CAD build for the part. Positions are in the model's coordinates, mm. A direction names the side the tool comes from. Give positions to 0.01 mm unless a question says otherwise; leave off trailing zeros. Order: outer loops, then holes, each group sorted by start corner. A loop starts at its lowest first (then second) coordinate and runs counter-clockwise, first axis right, second up.
Item 1: Band-saw the part on A-A on y = 4. Give the cut face in (x, z).
Item 2: Which spindle directions (+Z, -Z, +X, -X, +Y, -Y) get a long thin tool onto all of the face, cutting with end or side? Do faces 1 (the flat face through (-1, -5, 27.006)), 2 (the flat face through (-1, -6, 5)), 3 (the flat face through (-1, 18, 18)). Say none if no direction does.
Item 3: Flat gauge pins, fed straight in: P1, Ø8.5, axis at x = 1.5, z = 19, coming from the -Y side; P2, Ø11, axis at x = 20, z = 3.5, coming from the -Y side. Where does each tip first touch, or does it go through?
Item 4: Band-saw the part on C-C on y = -9. Give the cut face in (x, z).
Item 5: Band-saw the part on B-B on x = -20. Give the cut face in (y, z).
Item 6: Two-plate mould, pull along Z, no slides. Class faces 4 (the flat face through (-1, 0, 37)), 5 (the flat face through (65, 12, 22)), 6 (the flat face through (-1, 1, 10.006)): released by +Z, released by -Z, zero draft, split by the parting line, or undercut.
Item 7: Wall check: L1, parallel to Z at x = 2, y = 3.5; L2, parallel to Y at x = -53.5, z = 2; L3, parallel to Z at x = -49.5, y = -10.5. Give the ranges that are in metal, low to high.
Item 8: Band-saw the part on D-D on z = 22. Give the cut face in (x, y), plus the area to 3 significant figures.
```python
from build123d import *

# Parameters (mm, degrees)
SKETCH_2_W          = 130
SKETCH_2_H          = 36
EXTRUDE_1_DEPTH     = 37
CUT_EXTRUDE_START   = -18
SKETCH_4_W          = 130
SKETCH_4_H          = 17
CUT_EXTRUDE_1_DEPTH = 26
SKETCH_5_W          = 130
SKETCH_5_H          = 12
CUT_EXTRUDE_2_DEPTH = 12


with BuildPart() as part:
    # 스케치2 → 보스-돌출1 (new body)
    with BuildSketch(Plane.XY):
        Rectangle(SKETCH_2_W, SKETCH_2_H)
    extrude(amount=EXTRUDE_1_DEPTH)

    # 스케치4 → 컷-돌출1 (cut)
    with BuildSketch(Plane(origin=(0, 0, 0), x_dir=(1, 0, 0), z_dir=(0, 1, 0)).offset(CUT_EXTRUDE_START)):
        with Locations((0, -18.50644362)):
            Rectangle(SKETCH_4_W, SKETCH_4_H)
    extrude(amount=CUT_EXTRUDE_1_DEPTH, mode=Mode.SUBTRACT)

    # 스케치5 → 컷-돌출2 (cut)
    with BuildSketch(Plane(origin=(0, 0, 0), x_dir=(1, 0, 0), z_dir=(0, 1, 0)).offset(CUT_EXTRUDE_START)):
        with Locations((0, -6)):
            Rectangle(SKETCH_5_W, SKETCH_5_H)
    extrude(amount=CUT_EXTRUDE_2_DEPTH, mode=Mode.SUBTRACT)


solid = part.part
```
The answers:
1. outline: (-65, 0) - (65, 0) - (65, 10.01) - (-65, 10.01) - close; (-65, 27.01) - (65, 27.01) - (65, 37) - (-65, 37) - close
2. face 1: +X, -X, -Y
2. face 2: -Z, +X, -X, -Y
2. face 3: +Z, -Z, +X, -X, +Y
3. P1: stops at y = 8
3. P2: stops at y = -6
4. outline: (-65, 27.01) - (65, 27.01) - (65, 37) - (-65, 37) - close
5. outline: (-18, 27.01) - (8, 27.01) - (8, 10.01) - (-6, 10.01) - (-6, 0) - (18, 0) - (18, 37) - (-18, 37) - close
6. face 4: released by +Z
6. face 5: zero draft
6. face 6: undercut
7. L1: z = 0 to 10.01, 27.01 to 37
7. L2: y = -6 to 18
7. L3: z = 27.01 to 37
8. outline: (-65, 8) - (65, 8) - (65, 18) - (-65, 18) - close
8. area: 1,300 mm2
